The figure shows three views and two pictorial views of one solid part (mm, origin at its lowest corner). Answer the questions. Round coordinates to 2 decimals unless told otherwise and drop trailing zeros. Order: outer loops, then holes, each group sorted by start corner. A loop starts at its lowest first (then second) coordinate and runs counter-clockwise, first axis right, second up. Notation, with made-up numbers: (-16, 74.25) -> (7, 74.25) arc R10 ccw to (7, 80.25) -> close; hole circle Ø11 at (24, 60.25). An arc over 180 degrees is marked (long way). Return JSON: item names as keys, results as strings. Group by question number.
(1) Determine the mould class of the marked faces 1, 2, 3 and 4 for opening direction X: +X half, -X half, draft (parallel to the pull), parting line (faces both ways), or undercut.
(2) The part is cut by section B-B (y = 48.5). Determine the outline of the cut face in (x, z).
(3) The part is cut by section D-D (y = 9). Determine the outline of the cut face in (x, z).
(4) Consider line 1 (Y direction, x = 5, z = 1.05); line 2 (X direction, y = 48.5, z = 2); line 3 (Y direction, x = 5.75, z = 1.5). Determine where each line is inside the solid, lowest interval first. Write a range as [from, to].
(5) The part is cut by section C-C (x = 5). Determine the outline of the cut face in (y, z), plus the area to 3 significant figures.
(6) The part is cut by section A-A (z = 2.4). Determine the outline of the cut face in (x, y).
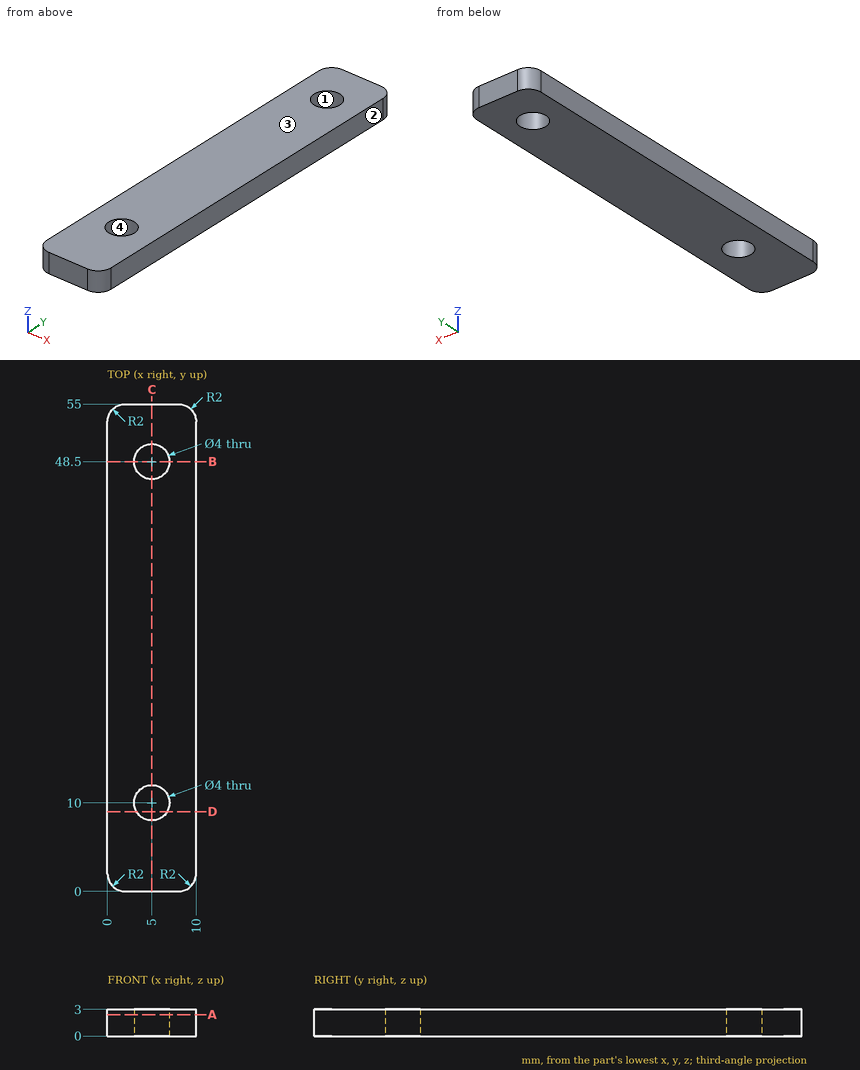
Answer below:
{
 "1": {"face 1": "undercut", "face 2": "+X half", "face 3": "draft", "face 4": "undercut"},
 "2": {"outline": "(0, 0) -> (3, 0) -> (3, 3) -> (0, 3) -> close; (7, 0) -> (10, 0) -> (10, 3) -> (7, 3) -> close"},
 "3": {"outline": "(0, 0) -> (3.27, 0) -> (3.27, 3) -> (0, 3) -> close; (6.73, 0) -> (10, 0) -> (10, 3) -> (6.73, 3) -> close"},
 "4": {"line 1": "y = [0, 8], [12, 46.5], [50.5, 55]", "line 2": "x = [0, 3], [7, 10]", "line 3": "y = [0, 8.15], [11.85, 46.65], [50.35, 55]"},
 "5": {"outline": "(0, 0) -> (8, 0) -> (8, 3) -> (0, 3) -> close; (12, 0) -> (46.5, 0) -> (46.5, 3) -> (12, 3) -> close; (50.5, 0) -> (55, 0) -> (55, 3) -> (50.5, 3) -> close", "area": "141 mm²"},
 "6": {"outline": "(0, 2) arc R2 ccw to (2, 0) -> (8, 0) arc R2 ccw to (10, 2) -> (10, 53) arc R2 ccw to (8, 55) -> (2, 55) arc R2 ccw to (0, 53) -> close; hole circle Ø4 at (5, 10); hole circle Ø4 at (5, 48.5)"}
}
